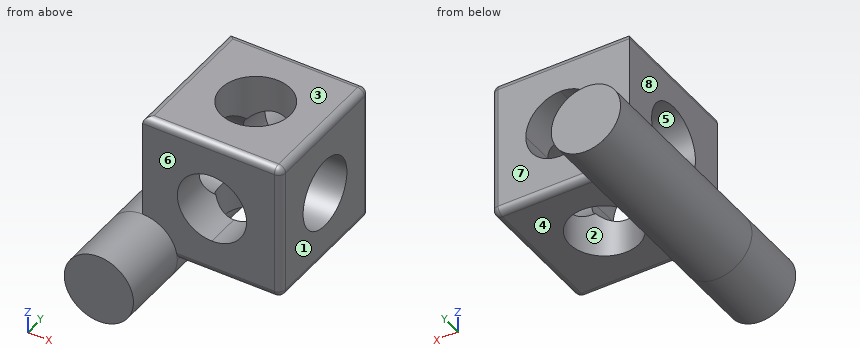
```python
from build123d import *

# Parameters (mm, degrees)
F0_W           = 101.6
F0_H           = 101.6
F1_DEPTH       = 101.6
F2_R           = 25.4
F3_DEPTH       = 101.6
F4_R           = 25.4
F5_DEPTH       = 101.6
F7_DEPTH       = 101.6
F8_R           = 5.08
F10_T1_DEPTH   = 91.44
F10_S5_W       = 5.08
F10_S5_H       = 5.08
F10_T6_DEPTH   = 5.08
F10_S11_W      = 5.08
F10_S11_H      = 5.08
F10_T12_DEPTH  = 5.08
F11_R          = 25.4
F12_DEPTH      = 50.8
F12_DEPTH_BACK = 152.4


# Not quite as in the source:
# - a fillet or chamfer that OpenCascade refuses, or shapes differently, is made with other operations: its cross-section is extruded or revolved along the edge and cut away or added


with BuildPart() as f1:
    # F0 (on Front) → F1 (new body)
    with BuildSketch(Plane.XZ):
        with Locations((50.8, 50.8)):
            Rectangle(F0_W, F0_H)
    extrude(amount=F1_DEPTH)

    # F2 (on face) → F3 (cut)
    with BuildSketch(Plane.XY.offset(101.6)):
        with Locations((50.8, -50.8)):
            Circle(F2_R)
    extrude(amount=-F3_DEPTH, mode=Mode.SUBTRACT)

    # F4 (on face) → F5 (cut)
    with BuildSketch(Plane(origin=(0, 0, 0), x_dir=(0, -1, 0), z_dir=(-1, 0, 0))):
        with Locations((50.8, 50.8)):
            Circle(F4_R)
    extrude(amount=-F5_DEPTH, mode=Mode.SUBTRACT)

    # F6 (on face) → F7 (cut)
    with BuildSketch(Plane.XZ.offset(101.6)):
        with BuildLine():
            ThreePointArc((76.2, 50.8), (68.7605122421, 68.7605122421), (50.8, 76.2))
            Line((50.8, 76.2), (50.8, 25.4))
            ThreePointArc((50.8, 25.4), (68.7605122421, 32.8394877579), (76.2, 50.8))
        make_face()
        with BuildLine():
            Line((50.8, 25.4), (50.8, 76.2))
            ThreePointArc((50.8, 76.2), (25.4, 50.8), (50.8, 25.4))
        make_face()
    extrude(amount=-F7_DEPTH, mode=Mode.SUBTRACT)

    # F8
    f8_edges = [f1.edges().sort_by_distance(p)[0] for p in [
        (50.8, -101.6, 101.6),
        (101.6, -50.8, 101.6),
        (50.8, 0, 101.6),
        (0, -50.8, 101.6),
        (101.6, -50.8, 0),
        (50.8, -101.6, 0),
        (0, -50.8, 0),
        (50.8, 0, 0),
        (101.6, 0, 50.8),
    ]]
    fillet(f8_edges, radius=F8_R)

    # F10: fillet of radius 5.08 on 1 edges, made by hand

    # F10_s2 → F10_t1 (cut)
    with BuildSketch(Plane.XY.offset(5.08)):
        with BuildLine():
            ThreePointArc((96.52, -101.6), (100.1121024484, -100.1121024484), (101.6, -96.52))
            Line((101.6, -96.52), (101.6, -101.6))
            Line((101.6, -101.6), (96.52, -101.6))
        make_face()
    extrude(amount=F10_T1_DEPTH, mode=Mode.SUBTRACT)


with BuildPart() as f10_tool4:
    # F10_s5 → F10_t6 (new body)
    with BuildSketch(Plane.XZ.offset(96.52)):
        with Locations((99.06, 2.54)):
            Rectangle(F10_S5_W, F10_S5_H)
    extrude(amount=F10_T6_DEPTH)

    # F10_s7 → F10_t8 (revolve, cut)
    with BuildSketch(Plane(origin=(96.52, -96.52, 5.08), x_dir=(-0.7071067812, 0, 0.7071067812), z_dir=(0.7071067812, 0, 0.7071067812))):
        with BuildLine():
            ThreePointArc((0, -5.08), (5.08, 0), (0, 5.08))
            Line((0, 5.08), (0, -5.08))
        make_face()
    revolve(axis=Axis((96.52, -96.52, 5.08), (0, -1, 0)), mode=Mode.SUBTRACT)


with BuildPart() as f1_1:
    add(f1.part)

    # F10_t3: cut F10_tool4
    add(f10_tool4.part, mode=Mode.SUBTRACT)


with BuildPart() as f10_tool10:
    # F10_s11 → F10_t12 (new body)
    with BuildSketch(Plane.XZ.offset(96.52)):
        with Locations((99.06, 99.06)):
            Rectangle(F10_S11_W, F10_S11_H)
    extrude(amount=F10_T12_DEPTH)

    # F10_s13 → F10_t14 (revolve, cut)
    with BuildSketch(Plane(origin=(96.52, -96.52, 96.52), x_dir=(-0.7071067812, 0, -0.7071067812), z_dir=(-0.7071067812, 0, 0.7071067812))):
        with BuildLine():
            ThreePointArc((0, -5.08), (5.08, 0), (0, 5.08))
            Line((0, 5.08), (0, -5.08))
        make_face()
    revolve(axis=Axis((96.52, -96.52, 96.52), (0, -1, 0)), mode=Mode.SUBTRACT)


with BuildPart() as f1_2:
    add(f1_1.part)

    # F10_t9: cut F10_tool10
    add(f10_tool10.part, mode=Mode.SUBTRACT)

    # F11 (on offset) → F12 (join, two sides)
    with BuildSketch(Plane.XZ.offset(101.6)) as f12_sk:
        Circle(F11_R)
    extrude(amount=F12_DEPTH)
    extrude(f12_sk.sketch, amount=-F12_DEPTH_BACK)


solid = f1_2.part
```
Geometry check sheet. Reference: the model listing, model coordinates, mm. Face numbers are marked on the shaded views. A direction names the side the tool comes from. Coordinates: 2 decimals unless noted, no trailing zeros. Order: outer loops, then holes, each group sorted by start corner. A loop starts at its lowest first (then second) coordinate and runs counter-clockwise, first axis right, second up. Notation, with made-up numbers: (7.25, -28.5) - (16.25, -28.5) arc R26 cw to (16.25, -14.5) - close; hole circle Ø5 at (79, 70.25). An arc over 180 degrees is marked (long way). Answer as a JSON object with one key per item and string values. Group by question number.
Item 1: Draft check along X on the marked faces 1, 2 and 3. Enter one of: +X half, -X half, draft (parallel to the pull), parting line (faces both ways), or undercut.
Item 2: Sectioned sample at B-B, the plane y = -39. Record the cut outline in (x, z), and give its area (3 significant figures).
Item 3: Depth check by flat-ended pin: pin 1 Ø12 at (y, z) = (-60.5, 35) entering from +X; pin 2 Ø10 at (x, y) = (11.5, 25) entering from +Z; pin 3 Ø6 at (x, y) = (6, -48) entering from -Z; pin 4 Ø1.5 at (x, z) = (71, 71.5) entering from -Y. Enter the tip coordinate at first touch or a pass-through.
Item 4: Sectioned sample at A-A, the plane x = 81. Record the cut outline in (y, z).
Item 5: Sectioned sample at D-D, the plane z = 65.5. Record the cut outline in (x, y).
Item 6: Scan lines: probe 1 along Y at (x, z) = (50, 87); probe 2 along X at (y, z) = (-50, 79); probe 3 along Z at (x, y) = (86, -55.5). Record each from-to range of solid material in increasing order.
Item 7: Tool access check on the marked faces 4, 5, 6, 7 and 8. Record the directions out of +Z, -Z, +X, -X, +Y, -Y that give a thin tool (end or side, any length) a straight path to the whole face; none if there is none.
Item 8: Sectioned sample at C-C, the plane y = -15.5. Record the cut outline in (x, z), and give its area (3 significant figures).
Resolved:
{
 "1": {"face 1": "+X half", "face 2": "undercut", "face 3": "draft"},
 "2": {"outline": "(0, 25.4) arc R25.4 ccw (long way) to (25.4, 0) - (28.31, 0) - (28.31, 28.31) - (0, 28.31) - close; (0, 73.29) - (28.31, 73.29) - (28.31, 101.6) - (5.08, 101.6) arc R5.08 ccw to (0, 96.52) - close; (73.29, 0) - (96.52, 0) arc R5.08 ccw to (101.6, 5.08) - (101.6, 28.31) - (73.29, 28.31) - close; (73.29, 73.29) - (101.6, 73.29) - (101.6, 96.52) arc R5.08 ccw to (96.52, 101.6) - (73.29, 101.6) - close", "area": "4,710 mm^2"},
 "3": {"pin 1": "through", "pin 2": "z = 24.55", "pin 3": "z = -25.22", "pin 4": "y = -101.6"},
 "4": {"outline": "(-101.6, 5.08) arc R5.08 ccw to (-96.52, 0) - (-5.08, 0) arc R5.08 ccw to (0, 5.08) - (0, 96.52) arc R5.08 ccw to (-5.08, 101.6) - (-96.52, 101.6) arc R5.08 ccw to (-101.6, 96.52) - close; hole circle Ø50.8 at (-50.8, 50.8)"},
 "5": {"outline": "(0, -101.6) - (30.09, -101.6) - (30.09, -71.51) - (0, -71.51) - close; (0, -30.09) - (30.09, -30.09) - (30.09, 0) - (0, 0) - close; (71.51, -101.6) - (96.52, -101.6) arc R5.08 ccw to (101.6, -96.52) - (101.6, -71.51) - (71.51, -71.51) - close; (71.51, -30.09) - (101.6, -30.09) - (101.6, -5.08) arc R5.08 ccw to (96.52, 0) - (71.51, 0) - close"},
 "6": {"probe 1": "-101.6 to -76.19, -25.41 to 0", "probe 2": "0 to 25.41, 76.19 to 101.6", "probe 3": "0 to 25.84, 75.76 to 101.6"},
 "7": {"face 4": "-Z, +X, +Y, -Y", "face 5": "+X, -X", "face 6": "+Z, +X, -Y", "face 7": "+Z, +X, +Y", "face 8": "+Z, -X, +Y, -Y"},
 "8": {"outline": "(0, 25.4) arc R25.4 ccw (long way) to (25.4, 0) - (96.52, 0) arc R5.08 ccw to (101.6, 5.08) - (101.6, 96.52) arc R5.08 ccw to (96.52, 101.6) - (5.08, 101.6) arc R5.08 ccw to (0, 96.52) - close; hole circle Ø50.8 at (50.8, 50.8)", "area": "9,800 mm^2"}
}
